Can you work these out from the model? Positions are in its coordinate system, mm. A direction names the side the tool comes from. Coordinates: 2 decimals unless noted, no trailing zeros. Order: outer loops, then holes, each group sorted by start corner. A loop starts at its lowest first (then second) coordinate and runs counter-clockwise, first axis right, second up. Notation, with made-up numbers: (58, -11) -> (101, -11) arc R17 cw to (101, 22) -> close; hole circle Ø3 at (43, 74). An arc over 180 degrees is marked (long way). Answer in a Markdown table with one row per item.
Solid Edge part; units mm, degrees
sketch "Sketch1" plane through (0, 0, 0) normal (0, -1, 0) x (1, 0, 0)
  circle A0 centre (0, 0) radius 6.35
  circle A1 centre (0, 0) radius 15.875
extrude "Protrusion1" add sketch "Sketch1" along normal mid plane 9.525
sketch "Sketch2" plane through (0, -4.7625, 0) normal (0, -1, 0) x (1, 0, 0)
  circle A0 centre (0, 9) radius 1.5
  circle A1 centre (9, 0) radius 1.5
  circle A2 centre (0, -9) radius 1.5
  circle A3 centre (-9, 0) radius 1.5
  circle A4 centre (-6.4772, 6.4772) radius 1.5
  circle A5 centre (6.364, 6.364) radius 1.5
  circle A6 centre (6.364, -6.364) radius 1.5
  circle A7 centre (-6.364, -6.364) radius 1.5
extrude "Cutout1" cut sketch "Sketch2" against normal up to surface (9.525 mm away)
sketch "Sketch3" plane through (0, 0, 0) normal (0, 0, 1) x (1, 0, 0)
  line L0 (-15.875, -2.3812) -> (-11.1125, -2.3812)
  line L1 (-11.1125, -2.3812) -> (-11.1125, -4.7625)
  line L2 (-11.1125, -4.7625) -> (-15.875, -4.7625)
  line L3 (-15.875, -4.7625) -> (-15.875, -2.3812)
  line L4 (-15.875, 2.3812) -> (-11.1125, 2.3812)
  line L5 (-11.1125, 2.3812) -> (-11.1125, 4.7625)
  line L6 (-11.1125, 4.7625) -> (-15.875, 4.7625)
  line L7 (-15.875, 4.7625) -> (-15.875, 2.3812)
  dimension "D1" = 15.875
revolve "RevolvedCutout1" cut sketch "Sketch3" angle 360 about axis through (0, 54.0067, 0) along (0, -1, 0)
(1) Suppose I cut it at A-A (z = 0). Count the separate pieces of the cut face and the enclosed holes in it, and give its area (3 significant figures).
Response values:
| item | result |
|---|---|
| separate pieces | 4 |
| enclosed holes | 0 |
| area | 78.9 mm2 |
(2) I need wall thicknesses on line 1 (Z direction, x = 0, y = 0.25) (3 decimals); line 2 (Y direction, x = 13, z = 8.5); line 3 (Z direction, x = -3, y = 0.75). Which ranges of each line are inside material? Lowest first, please. Write a range as [from, to].
Response values:
| item | result |
|---|---|
| line 1 | [-15.875, -10.5], [-7.5, -6.35], [6.35, 7.5], [10.5, 15.875] |
| line 2 | [-2.38, 2.38] |
| line 3 | [-15.59, -5.6], [5.6, 15.59] |
(3) We'd pull the mould along Z, two halves only. Please class faces 4 (the flat face through (-5, 4.762, -5)), 5 (the cylindrical face through (-1.38, 0.07, 6.2)), 6 (the cylindrical face through (-0.325, -0.067, 7.536)), 7 (the cylindrical face through (-10.6, -3.59, -3.34)): +Z half, -Z half, draft (parallel to the pull), parting line (faces both ways), or undercut.
Response values:
| item | result |
|---|---|
| face 4 | draft |
| face 5 | undercut |
| face 6 | undercut |
| face 7 | parting line |
(4) Suppose I cut it at D-D (x = 9). Please give me the cut outline in (y, z), and give its area (3 significant figures).
Response values:
| item | result |
|---|---|
| outline | (-4.76, -6.52) -> (-2.38, -6.52) -> (-2.38, -13.08) -> (2.38, -13.08) -> (2.38, -6.52) -> (4.76, -6.52) -> (4.76, -1.5) -> (-4.76, -1.5) -> close; (-4.76, 1.5) -> (4.76, 1.5) -> (4.76, 6.52) -> (2.38, 6.52) -> (2.38, 13.08) -> (-2.38, 13.08) -> (-2.38, 6.52) -> (-4.76, 6.52) -> close |
| area | 158 mm2 |
(5) On a 3-axis mill with a long thin cutter (end or side, diameter ignored), from which of +Z, -Z, +X, -X, +Y, -Y can I reach the whole of each face in a straight line? I mean faces 1 (the flat face through (11, -2.381, 3)), 2 (the cylindrical face through (-10.6, 3.59, 3.34)), 3 (the cylindrical face through (7.17, -0.07, 7.63)). Say none if no direction works.
Response values:
| item | result |
|---|---|
| face 1 | -Y |
| face 2 | +Y |
| face 3 | +Y, -Y |
(6) Will these pins go through, and if not, where does the flat tip stop? pin 1 Ø4 at (x, y) = (-9.5, 1.5) entering from +Z; pin 2 Ø1.8 at (x, z) = (-6.364, -6.364) entering from +Y; pin 3 Ø5 at (y, z) = (2, 11.5) entering from -X.
Response values:
| item | result |
|---|---|
| pin 1 | z = 13.99 |
| pin 2 | through |
| pin 3 | x = -13.08 |
(7) Suppose I cut it at C-C (z = -10). Please give me the cut outline in (x, y).
Response values:
| item | result |
|---|---|
| outline | (-12.33, -2.38) -> (-4.85, -2.38) -> (-4.85, -4.76) -> (-1.12, -4.76) -> (-1.12, 4.76) -> (-4.85, 4.76) -> (-4.85, 2.38) -> (-12.33, 2.38) -> close; (1.12, -4.76) -> (4.85, -4.76) -> (4.85, -2.38) -> (12.33, -2.38) -> (12.33, 2.38) -> (4.85, 2.38) -> (4.85, 4.76) -> (1.12, 4.76) -> close |
